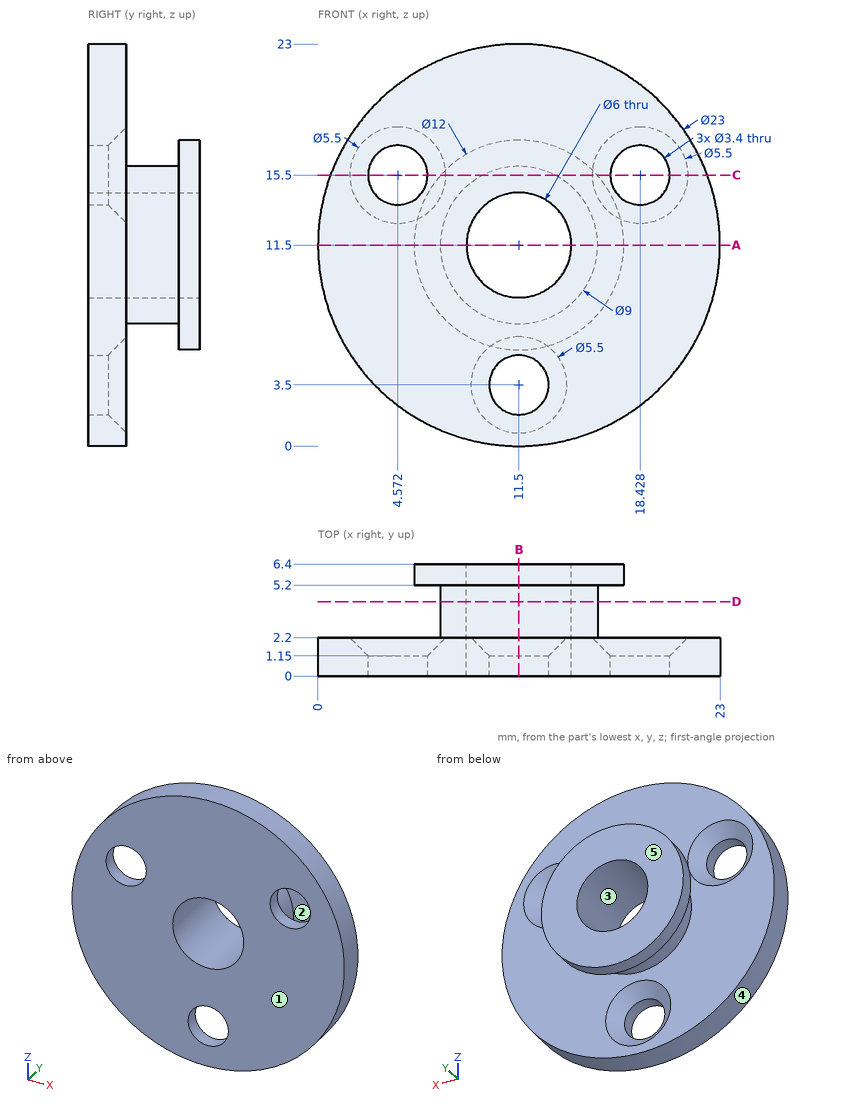
Could you check a few things on this drawing? It's one solid part, dimensions in mm from its lowest x, y, z. A direction names the side the tool comes from. Give positions to 0.01 mm unless a question says otherwise; leave off trailing zeros. Write each loop counter-clockwise with the first axis right and the second up, starting at its lowest first coordinate (ties: lowest second). Pieces come first, ordered by that corner, then holes. Notation, with made-up numbers: (20.5, -35) -> (29.5, -35) arc R19 ccw to (29.5, -28) -> close; hole circle Ø3 at (72.5, 36). An arc over 180 degrees is marked (long way). Write each question's results on one line, items separated by ' | '.
1. I want a section at A-A, the plane z = 11.5. Write out the boundary of the cut face in (x, y).
Check sheet entries:
outline: (0, 0) -> (8.5, 0) -> (8.5, 6.4) -> (5.5, 6.4) -> (5.5, 5.2) -> (7, 5.2) -> (7, 2.2) -> (0, 2.2) -> close; (14.5, 0) -> (23, 0) -> (23, 2.2) -> (16, 2.2) -> (16, 5.2) -> (17.5, 5.2) -> (17.5, 6.4) -> (14.5, 6.4) -> close
2. On a 3-axis mill with a long thin cutter (end or side, diameter ignored), from which of +Z, -Z, +X, -X, +Y, -Y can I reach the whole of each face in a straight line? I mean the marked faces 1 and 2. Say none if no direction works.
Check sheet entries:
face 1: +Z, -Z, +X, -X, -Y | face 2: none
3. I want a section at B-B, the plane x = 11.5. Write out the boundary of the cut face in (y, z), then the cut area to 3 significant figures.
Check sheet entries:
outline: (0, 0) -> (2.2, 0) -> (2.2, 0.75) -> (1.15, 1.8) -> (0, 1.8) -> close; (0, 5.2) -> (1.15, 5.2) -> (2.2, 6.25) -> (2.2, 7) -> (5.2, 7) -> (5.2, 5.5) -> (6.4, 5.5) -> (6.4, 8.5) -> (0, 8.5) -> close; (0, 14.5) -> (6.4, 14.5) -> (6.4, 17.5) -> (5.2, 17.5) -> (5.2, 16) -> (2.2, 16) -> (2.2, 23) -> (0, 23) -> close | area: 45.0 mm²
4. Will these pins go through, and if not, where does the flat tip stop? pin 1 Ø1 at (x, y) = (13, 2.5) entering from +Z; pin 2 Ø2 at (y, z) = (1, 14.5) entering from -X (1 decimal); pin 3 Ø1.5 at (x, y) = (15, 5) entering from +Z.
Check sheet entries:
pin 1: stops at z = 22.95 | pin 2: stops at x = 0.2 | pin 3: stops at z = 16.82
5. I need wall thicknesses on L1, parallel to X at y = 1.5, z = 11.5; L2, parallel to X at y = 0.2, z = 15.5; L3, parallel to Y at x = 6.75, z = 10.5. Which ranges of each line are inside material? Lowest first, please.
Check sheet entries:
L1: x = 0 to 8.5, 14.5 to 23 | L2: x = 0.72 to 2.87, 6.27 to 16.73, 20.13 to 22.28 | L3: y = 0 to 2.2, 5.2 to 6.4
6. I want a section at D-D, the plane y = 4.25. Write out the boundary of the cut face in (x, z).
Check sheet entries:
outline: circle Ø9 at (11.5, 11.5); hole circle Ø6 at (11.5, 11.5)
7. I want a section at C-C, the plane z = 15.5. Write out the boundary of the cut face in (x, y), then the cut area to 3 significant figures.
Check sheet entries:
outline: (0.72, 0) -> (2.87, 0) -> (2.87, 1.15) -> (1.82, 2.2) -> (0.72, 2.2) -> close; (6.27, 0) -> (16.73, 0) -> (16.73, 1.15) -> (15.68, 2.2) -> (13.56, 2.2) -> (13.56, 5.2) -> (15.97, 5.2) -> (15.97, 6.4) -> (7.03, 6.4) -> (7.03, 5.2) -> (9.44, 5.2) -> (9.44, 2.2) -> (7.32, 2.2) -> (6.27, 1.15) -> close; (20.13, 0) -> (22.28, 0) -> (22.28, 2.2) -> (21.18, 2.2) -> (20.13, 1.15) -> close | area: 53.4 mm²
8. If we mould it in two halves opening along X, with no side actions, what happens to the marked faces 3, 4 and 5? For each: released by +X, released by -X, zero draft, split by the parting line, or undercut.
Check sheet entries:
face 3: undercut | face 4: split by the parting line | face 5: zero draft
